Could you check a few things on this model? Use its own coordinates, in mm. Round coordinates to 2 decimals unless told otherwise and drop trailing zeros. Write each loop counter-clockwise with the first axis right and the second up, starting at its lowest first coordinate (ties: lowest second). Pieces come first, ordered by that corner, then holes. Notation, with made-up numbers: (70.5, 54.5) -> (128.5, 54.5) arc R27 cw to (128.5, 89.5) -> close; hole circle Ø1 at (-34, 66.5). An arc over 180 degrees is marked (long way). Answer in a Markdown table with one row per item.
Autodesk Inventor part; units mm, degrees
ref_plane "YZ Plane" through (0, 0, 0) normal (1, 0, 0) x (0, 1, 0)
ref_plane "XZ Plane" through (0, 0, 0) normal (0, 1, 0) x (-1, 0, 0)
ref_plane "XY Plane" through (0, 0, 0) normal (0, 0, 1) x (1, 0, 0)
sketch "Sketch2" plane through (0, 0, 0) normal (0, 0, 1) x (1, 0, 0)
  circle A0 centre (0, 0) radius 45.5
  circle A1 centre (0, 0) radius 95
  dimension "d25" = 91
  dimension "d27" = 190
extrude "Plate2" add sketch "Sketch2" along normal blind 8
sketch "Sketch3" plane through (0, 0, 8) normal (0, 0, 1) x (1, 0, 0)
  circle A0 centre (-80, 0) radius 8.5
  circle A1 centre (0, 0) radius 80 construction
  dimension "d28" = 160
  dimension "d15" = 17
extrude "Cut1" cut sketch "Sketch3" against normal blind 8
pattern_circular "Circular Pattern1" count 4 over 360 about axis through (0, 0, -10) along (0, 0, 1) of "Cut1"
equation "\"d17\" = Thickness"
equation "\"d14\" = Thickness"
equation "\"BendReliefWidth\" = Thickness"
equation "\"BendReliefDepth\" = 0.5 * Thickness"
equation "\"CornerReliefSize\" = 4 * Thickness"
equation "\"MinimumRemnant\" = 2 * Thickness"
equation "\"TransitionRadius\" = BendRadius"
equation "\"JacobiRadiusSize\" = BendRadius"
equation "\"GapSize\" = Thickness"
properties part number "PNS 734 FDS flange DN90" material "Steel"
1) Thinking about a two-plate mould opening in Y: for faces 1 (the face through (41, 22, 8)), 2 (the face through (-20.59, 92.74, 3.94)), 3 (the face through (0.37, 88.49, 4.06)), which applies, +Y half, -Y half, draft (parallel to the pull), parting line (faces both ways), or undercut?
Findings:
| item | result |
|---|---|
| face 1 | draft |
| face 2 | parting line |
| face 3 | undercut |
2) Imagine slicing it at A-A, the plane y = 0. Please give me the cut outline in (x, z), plus the area to 3 significant figures.
Findings:
| item | result |
|---|---|
| outline | (-95, 0) -> (-88.5, 0) -> (-88.5, 8) -> (-95, 8) -> close; (-71.5, 0) -> (-45.5, 0) -> (-45.5, 8) -> (-71.5, 8) -> close; (45.5, 0) -> (71.5, 0) -> (71.5, 8) -> (45.5, 8) -> close; (88.5, 0) -> (95, 0) -> (95, 8) -> (88.5, 8) -> close |
| area | 520 mm^2 |
3) Imagine slicing it at C-C, the plane z = 1.5. Please give me the cut outline in (x, y).
Findings:
| item | result |
|---|---|
| outline | circle Ø190 at (0, 0); hole circle Ø17 at (-80, 0); hole circle Ø91 at (0, 0); hole circle Ø17 at (0, -80); hole circle Ø17 at (0, 80); hole circle Ø17 at (80, 0) |
4) For pin 1 (3 mm diameter, centred on y = -8, z = 4.5, fed in from -X); pin 2 (19.5 mm diameter, centred on x = 0, y = -80, fed in from +Z); pin 3 (4 mm diameter, centred on x = -11.5, z = 3, fed in from -Y); pin 4 (4 mm diameter, centred on y = 65.5, z = 1, fed in from +X), each with a flat end and sliding along its axis, tell me the tip position at first contact or that it passes through.
Findings:
| item | result |
|---|---|
| pin 1 | stops at x = -94.78 |
| pin 2 | stops at z = 8 |
| pin 3 | stops at y = -94.52 |
| pin 4 | stops at x = 70.66 |
5) Imagine slicing it at D-D, the plane x = -80. Please give me the cut outline in (y, z).
Findings:
| item | result |
|---|---|
| outline | (-51.23, 0) -> (-8.5, 0) -> (-8.5, 8) -> (-51.23, 8) -> close; (8.5, 0) -> (51.23, 0) -> (51.23, 8) -> (8.5, 8) -> close |
6) Please list where these lines run through material, in increasing order: line 1 (X direction, y = -0.5, z = 4.5); line 2 (Y direction, x = 7, z = 1); line 3 (X direction, y = -13.5, z = 0.5).
Findings:
| item | result |
|---|---|
| line 1 | x = -95 to -88.49, -71.51 to -45.5, 45.5 to 71.51, 88.49 to 95 |
| line 2 | y = -94.74 to -84.82, -75.18 to -44.96, 44.96 to 75.18, 84.82 to 94.74 |
| line 3 | x = -94.04 to -43.45, 43.45 to 94.04 |
